The model under review builds one solid part; all positions refer to its coordinate system, in mm. Face numbers are marked on the shaded views. A direction names the side the tool comes from. Give positions to 0.01 mm unless a question says otherwise; leave off trailing zeros. Order: outer loops, then holes, each group sorted by start corner. A loop starts at its lowest first (then second) coordinate and runs counter-clockwise, first axis right, second up.
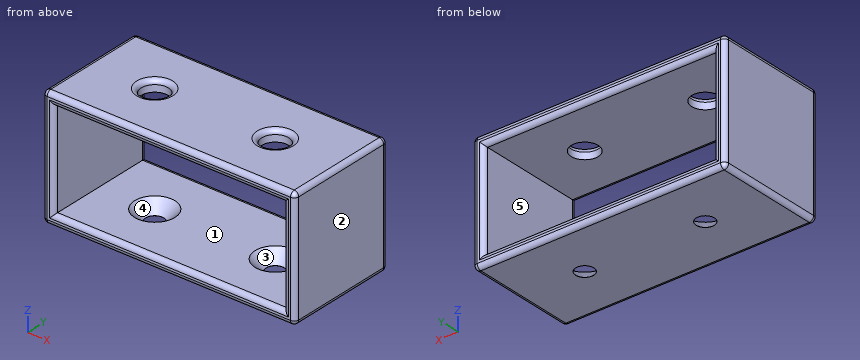
```python
from build123d import *

# Parameters (mm, degrees)
SKETCH_W          = 56
SKETCH_H          = 26.5
PAD_DEPTH         = 25
SKETCH001_W       = 51
SKETCH001_H       = 21.5
POCKET_DEPTH      = 0.001
POCKET_DEPTH_BACK = 25.001
SKETCH002_R       = 3
POCKET001_DEPTH   = 3.5
SKETCH003_R       = 2
POCKET002_DEPTH   = 2.5
CHAMFER_SIZE      = 2.485
FILLET_R          = 1


with BuildPart() as part:
    # Sketch → Pad (new body)
    with BuildSketch(Plane.XZ):
        Rectangle(SKETCH_W, SKETCH_H)
    extrude(amount=PAD_DEPTH)

    # Sketch001 → Pocket (cut, two sides)
    with BuildSketch(Plane.XZ) as pocket_sk:
        Rectangle(SKETCH001_W, SKETCH001_H)
    extrude(amount=-POCKET_DEPTH, mode=Mode.SUBTRACT)
    extrude(pocket_sk.sketch, amount=POCKET_DEPTH_BACK, mode=Mode.SUBTRACT)

    # Sketch002 (on DatumPlane) → Pocket001 (cut)
    with BuildSketch(Plane(origin=(0, 0, 13.25), x_dir=(-1, 0, 0), z_dir=(0, 0, 1))):
        with Locations((-13.375, 12.5)):
            Circle(SKETCH002_R)
        with Locations((13.375, 12.5)):
            Circle(SKETCH002_R)
    extrude(amount=-POCKET001_DEPTH, mode=Mode.SUBTRACT)

    # Sketch003 (on DatumPlane) → Pocket002 (cut)
    with BuildSketch(Plane(origin=(0, 0, -10.75), x_dir=(-1, 0, 0), z_dir=(0, 0, 1))):
        with Locations((-13.375, 12.5)):
            Circle(SKETCH003_R)
        with Locations((13.375, 12.5)):
            Circle(SKETCH003_R)
    extrude(amount=-POCKET002_DEPTH, mode=Mode.SUBTRACT)

    # Chamfer
    chamfer_edges = [part.edges().sort_by_distance(p)[0] for p in [
        (-11.375, -12.5, -10.75),
        (15.375, -12.5, -10.75),
    ]]
    chamfer(chamfer_edges, length=CHAMFER_SIZE)

    # Fillet
    fillet_edges = [part.edges().sort_by_distance(p)[0] for p in [
        (-28, -25, 0),
        (0, -25, 13.25),
        (0, -25, -13.25),
        (28, -25, 0),
        (-25.5, -25, 0),
        (0, -25, 10.75),
        (25.5, -25, 0),
        (0, -25, -10.75),
        (-28, 0, 0),
        (0, 0, 13.25),
        (0, 0, -13.25),
        (28, 0, 0),
        (-25.5, 0, 0),
        (0, 0, 10.75),
        (25.5, 0, 0),
        (0, 0, -10.75),
        (28, -12.5, 13.25),
        (28, -12.5, -13.25),
        (-28, -12.5, -13.25),
        (-28, -12.5, 13.25),
        (16.375, -12.5, 13.25),
        (-10.375, -12.5, 13.25),
    ]]
    fillet(fillet_edges, radius=FILLET_R)


solid = part.part
```
Item 1: Draft analysis for pull direction Y (two halves, no side actions). For the marked faces 4 and 5, state which applies: released by +Y, released by -Y, zero draft, split by the parting line, or undercut.
Values found:
face 4: undercut
face 5: zero draft
Item 2: For line 1 (X direction, y = -12.5, z = 11.75) (3 decimals); line 2 (Z direction, x = -24, y = -10.25); line 3 (X direction, y = -11.5, z = -9.5), list the stretches that pass through material, from the lowest coordinate up.
Values found:
line 1: x = -28 to -16.375, -10.375 to 10.375, 16.375 to 28
line 2: z = -13.25 to -10.75, 10.75 to 13.25
line 3: x = -28 to -25.5, 25.5 to 28
Item 3: For the marked faces 1, 2 and 3, list the 3-axis set-ups (+Z, -Z, +X, -X, +Y, -Y) from which the entire face can be reached by the end or side of a thin tool; tool diameter is ignored.
Values found:
face 1: +Y, -Y
face 2: +Z, -Z, +X, +Y, -Y
face 3: none
Item 4: Take a section at A-A (y = -20). Give the boundary of the cut face in (x, z), and give its area (3 significant figures).
Values found:
outline: (-28, -12.25) arc R1 ccw to (-27, -13.25) - (27, -13.25) arc R1 ccw to (28, -12.25) - (28, 12.25) arc R1 ccw to (27, 13.25) - (-27, 13.25) arc R1 ccw to (-28, 12.25) - close; hole (-25.5, -10.75) - (25.5, -10.75) - (25.5, 10.75) - (-25.5, 10.75) - close
area: 387 mm2
Item 5: Clearance check with a flat-ended pin moving along its axis: pin 1 Ø2.5 at (x, y) = (13.375, -12.5) entering from +Z. State where the tip first meets the part, or that it passes through.
Values found:
pin 1: passes through
Item 6: Take a section at D-D (y = -12.5). Give the number of separate pieces and of enclosed holes in the cut face, and give its area (3 significant figures).
Values found:
separate pieces: 4
enclosed holes: 0
area: 323 mm2
Item 7: Take a section at C-C (z = 6.5). Give the boundary of the cut face in (x, y), and give its area (3 significant figures).
Values found:
outline: (-28, -24) arc R1 ccw to (-27, -25) - (-26.5, -25) arc R1 ccw to (-25.5, -24) - (-25.5, -1) arc R1 ccw to (-26.5, 0) - (-27, 0) arc R1 ccw to (-28, -1) - close; (25.5, -24) arc R1 ccw to (26.5, -25) - (27, -25) arc R1 ccw to (28, -24) - (28, -1) arc R1 ccw to (27, 0) - (26.5, 0) arc R1 ccw to (25.5, -1) - close
area: 123 mm2
Item 8: Take a section at B-B (x = -19.5). Give the boundary of the cut face in (y, z).
Values found:
outline: (-25, -12.25) arc R1 ccw to (-24, -13.25) - (-1, -13.25) arc R1 ccw to (0, -12.25) - (0, -11.75) arc R1 ccw to (-1, -10.75) - (-24, -10.75) arc R1 ccw to (-25, -11.75) - close; (-25, 11.75) arc R1 ccw to (-24, 10.75) - (-1, 10.75) arc R1 ccw to (0, 11.75) - (0, 12.25) arc R1 ccw to (-1, 13.25) - (-24, 13.25) arc R1 ccw to (-25, 12.25) - close
